Verification items for the finished model (mm, model axes). A direction names the side the tool comes from. Give positions to 0.01 mm unless a question says otherwise; leave off trailing zeros. Write each loop counter-clockwise with the first axis right and the second up, starting at its lowest first coordinate (ties: lowest second). Pieces come first, ordered by that corner, then holes. Notation, with made-up numbers: (67.5, 69.5) - (88.5, 69.5) arc R8 cw to (88.5, 80.5) - close; hole circle Ø4 at (44.5, 54.25). An arc over 180 degrees is marked (long way). Answer as a JSON object with one key per item and string values. Group by question number.
Item 1: Sectioned sample at B-B, the plane z = 3. Record the boundary of the cut face in (x, y), and give its area (3 significant figures).
Item 2: Sectioned sample at C-C, the plane y = 27. Record the boundary of the cut face in (x, z).
Item 3: Draft check along Y on faces 1 (the face through (-56, 28, -4.278)), 2 (the face through (-53.159, 28, 1)), 3 (the face through (-55, 33.099, 1)). Enter one of: +Y half, -Y half, draft (parallel to the pull), parting line (faces both ways), or undercut.
Item 4: Sectioned sample at D-D, the plane z = 0.5. Record the boundary of the cut face in (x, y).
Item 5: Scan lines: line 1 along Y through (x, z) = (-54.5, -2.5); line 2 along X through (y, z) = (26, -1.75); line 3 along X through (y, z) = (28, 0). Record each from-to range of solid material in increasing order. Write a range as [from, to].
Item 6: Tool access check on faces 4 (the face through (-57.008, 26.689, 1.442)), 5 (the face through (-54, 31.16, 1)), 6 (the face through (-55, 23.099, 1)). Record the directions out of +Z, -Z, +X, -X, +Y, -Y that give a thin tool (end or side, any length) a straight path to the whole face; none if there is none.
Item 7: Sectioned sample at A-A, the plane x = -53.5. Record the boundary of the cut face in (y, z).
```python
from build123d import *

# Parameters (mm, degrees)
SKETCH038_W             = 10
SKETCH038_H             = 10
PAD014_DEPTH            = 8
SKETCH039_R             = 1.45
POCKET009_DEPTH         = 5
SKETCH040_W             = 6.2
SKETCH040_H             = 1.8
POCKET010_DEPTH         = 15
BODY015_PLACEMENT_ANGLE = 90


with BuildPart() as part:
    # Sketch038 → Pad014 (new body)
    with BuildSketch(Plane.XY):
        with Locations((0.72243, -0.901424)):
            Rectangle(SKETCH038_W, SKETCH038_H)
    extrude(amount=PAD014_DEPTH)

    # Sketch039 (on Face6 of Pad014) → Pocket009 (cut)
    with BuildSketch(Plane.XY.offset(8)):
        with Locations((0.772802, -1.024983)):
            Circle(SKETCH039_R)
    extrude(amount=-POCKET009_DEPTH, mode=Mode.SUBTRACT)

    # Sketch040 (on Face2 of Pocket009) → Pocket010 (cut)
    with BuildSketch(Plane(origin=(-4.27757, 0, 0), x_dir=(0, -1, 0), z_dir=(-1, 0, 0))):
        with Locations((0.940135, 3.059345)):
            Rectangle(SKETCH040_W, SKETCH040_H)
    extrude(amount=-POCKET010_DEPTH, mode=Mode.SUBTRACT)


with BuildPart() as part_1:
    # Body015 placement: moved
    add(part.part.moved(Location((-51, 29, 0))).rotate(Axis((-51, 29, 0), (0, -1, 0)), BODY015_PLACEMENT_ANGLE))


solid = part_1.part
```
Geometry check:
{
 "1": {"outline": "(-59, 23.1) - (-51, 23.1) - (-51, 33.1) - (-59, 33.1) - close; hole (-54.96, 24.96) - (-53.16, 24.96) - (-53.16, 31.16) - (-54.96, 31.16) - close", "area": "68.8 mm^2"},
 "2": {"outline": "(-59, -4.28) - (-54.96, -4.28) - (-54.96, -0.3) - (-59, -0.3) - close; (-59, 1.85) - (-54.96, 1.85) - (-54.96, 5.72) - (-59, 5.72) - close; (-53.16, -4.28) - (-51, -4.28) - (-51, 5.72) - (-53.16, 5.72) - close"},
 "3": {"face 1": "draft", "face 2": "undercut", "face 3": "+Y half"},
 "4": {"outline": "(-59, 23.1) - (-51, 23.1) - (-51, 33.1) - (-59, 33.1) - (-59, 29.4) - (-54.96, 29.4) - (-54.96, 31.16) - (-53.16, 31.16) - (-53.16, 24.96) - (-54.96, 24.96) - (-54.96, 26.55) - (-59, 26.55) - close"},
 "5": {"line 1": "[23.1, 24.96], [31.16, 33.1]", "line 2": "[-59, -54.96], [-53.16, -51]", "line 3": "[-53.16, -51]"},
 "6": {"face 4": "-X", "face 5": "+Z, -Z", "face 6": "+Z, -Z, +X, -X, -Y"},
 "7": {"outline": "(23.1, -4.28) - (24.96, -4.28) - (24.96, 5.72) - (23.1, 5.72) - close; (31.16, -4.28) - (33.1, -4.28) - (33.1, 5.72) - (31.16, 5.72) - close"}
}
